Check sheet for the modelled part. Datum: model origin and axes. Units: mm. A direction names the side the tool comes from. Round coordinates to 2 decimals unless told otherwise and drop trailing zeros. Loops run counter-clockwise (first coordinate to the right, second up) from the corner with the lowest first, then second, coordinate; pieces in that order, holes last. Notation, with made-up numbers: (40, 13) -> (47, 13) arc R30 ccw to (47, 50) -> close; hole circle Ø7 at (-23, -38.5). An arc over 180 degrees is marked (long way). One line per question, with ' | ' between items.
```python
from build123d import *

# Parameters (mm, degrees)
F1_DEPTH = 42
F3_DEPTH = 18
F4_W     = 10.5735106468
F4_H     = 30
F4_W_2   = 10.8430571854
F5_DEPTH = 19
F7_DEPTH = 10
F9_D     = 5.5


with BuildPart() as f1:
    # F0 (on Front) → F1 (new body)
    with BuildSketch(Plane.XZ):
        Polygon((-16.5, -30), (-3.5, -30), (-3.5, -12), (16.5, -12), (16.5, 30), (-2.5, 30), (-2.5, 0), (-16.5, 0), align=None)
    extrude(amount=F1_DEPTH)

    # F2 (on face) → F3 (cut)
    with BuildSketch(Plane(origin=(0, 0, -30), x_dir=(1, 0, 0), z_dir=(0, 0, -1))):
        with BuildLine():
            Line((-3.5, 0.1923091142), (-3.5, 41.8076908858))
            ThreePointArc((-3.5, 41.8076908858), (-12.3, 21), (-3.5, 0.1923091142))
        make_face()
    extrude(amount=-F3_DEPTH, mode=Mode.SUBTRACT)

    # F4 (on face) → F5 (cut, through all)
    with BuildSketch(Plane.YZ.offset(16.5)):
        with Locations((-36.7132446766, 15)):
            Rectangle(F4_W, F4_H)
        with Locations((-5.4215285927, 15)):
            Rectangle(F4_W_2, F4_H)
    extrude(amount=-F5_DEPTH, mode=Mode.SUBTRACT)

    # F6 (on face) → F7 (cut)
    with BuildSketch(Plane.YZ.offset(16.5)):
        with BuildLine():
            Line((-15.8430571854, 30), (-26.4264893532, 30))
            Line((-26.4264893532, 30), (-26.4264893532, 3))
            ThreePointArc((-26.4264893532, 3), (-25.5478096967, 0.8786796564), (-23.4264893532, 0))
            Line((-23.4264893532, 0), (-18.8430571854, 0))
            ThreePointArc((-18.8430571854, 0), (-16.7217368419, 0.8786796564), (-15.8430571854, 3))
            Line((-15.8430571854, 3), (-15.8430571854, 30))
        make_face()
    extrude(amount=-F7_DEPTH, mode=Mode.SUBTRACT)

    # F9 (through all)
    with Locations(Plane.YZ.offset(6.5)):
        with Locations((-20.8430571854, 25), (-20.8430571854, 16)):
            Hole(F9_D / 2)


solid = f1.part
```
(1) Mould release check, pull along Y, two halves, no side actions. Record for faces 1 (the face through (12, -26.426, 17)), 2 (the face through (-13, -21, -30)), 3 (the face through (-4, 0, -11)): +Y half, -Y half, draft (parallel to the pull), parting line (faces both ways), or undercut.
Answer:
face 1: undercut | face 2: draft | face 3: +Y half
(2) Scan lines: probe 1 along Z at (x, y) = (-5.5, -9); probe 2 along Z at (x, y) = (6, -20); probe 3 along Z at (x, y) = (-11, -33.5). Record each from-to range of solid material in increasing order.
Answer:
probe 1: z = -12 to 0 | probe 2: z = -12 to 13.38, 18.62 to 22.38, 27.62 to 30 | probe 3: z = -30 to 0
(3) Sectioned sample at C-C, the plane y = -21.5. Record the cut outline in (x, z).
Answer:
outline: (-16.5, -30) -> (-12.3, -30) -> (-12.3, -12) -> (16.5, -12) -> (16.5, 0) -> (6.5, 0) -> (6.5, 13.33) -> (-2.5, 13.33) -> (-2.5, 0) -> (-16.5, 0) -> close; (-2.5, 18.67) -> (6.5, 18.67) -> (6.5, 22.33) -> (-2.5, 22.33) -> close; (-2.5, 27.67) -> (6.5, 27.67) -> (6.5, 30) -> (-2.5, 30) -> close
(4) Go/stop test with flat-tipped pins: pin 1 (10 mm diameter, centred on x = -5.5, z = 9, fed in from -Y); pin 2 (10 mm diameter, centred on x = -8, y = -5, fed in from +Z); pin 3 (6 mm diameter, centred on y = -30.5, z = 6, fed in from -X). Record where each tip stops, or that it passes through.
Answer:
pin 1: stops at y = -31.43 | pin 2: stops at z = 0 | pin 3: stops at x = -2.5
(5) Sectioned sample at B-B, the plane x = 3. Record the cut outline in (y, z).
Answer:
outline: (-42, -12) -> (0, -12) -> (0, 0) -> (-10.84, 0) -> (-10.84, 30) -> (-31.43, 30) -> (-31.43, 0) -> (-42, 0) -> close; hole circle Ø5.5 at (-20.84, 16); hole circle Ø5.5 at (-20.84, 25)
(6) Set-up check for faces 4 (the face through (-2.5, -21, 12)), 5 (the face through (7, -31.426, 15)), 6 (the face through (7, -10.843, 15)): record each of +Z, -Z, +X, -X, +Y, -Y from which the full face is reachable in a straight line by a thin tool's end or side.
Answer:
face 4: +Z, -X, +Y, -Y | face 5: +Z, +X, -X, -Y | face 6: +Z, +X, -X, +Y
(7) Sectioned sample at A-A, the plane z = 16. Record the cut outline in (x, y).
Answer:
outline: (-2.5, -31.43) -> (16.5, -31.43) -> (16.5, -26.43) -> (6.5, -26.43) -> (6.5, -23.59) -> (-2.5, -23.59) -> close; (-2.5, -18.09) -> (6.5, -18.09) -> (6.5, -15.84) -> (16.5, -15.84) -> (16.5, -10.84) -> (-2.5, -10.84) -> close
(8) Sectioned sample at D-D, the plane x = 9.5. Record the cut outline in (y, z).
Answer:
outline: (-42, -12) -> (0, -12) -> (0, 0) -> (-10.84, 0) -> (-10.84, 30) -> (-15.84, 30) -> (-15.84, 3) arc R3 cw to (-18.84, 0) -> (-23.43, 0) arc R3 cw to (-26.43, 3) -> (-26.43, 30) -> (-31.43, 30) -> (-31.43, 0) -> (-42, 0) -> close
